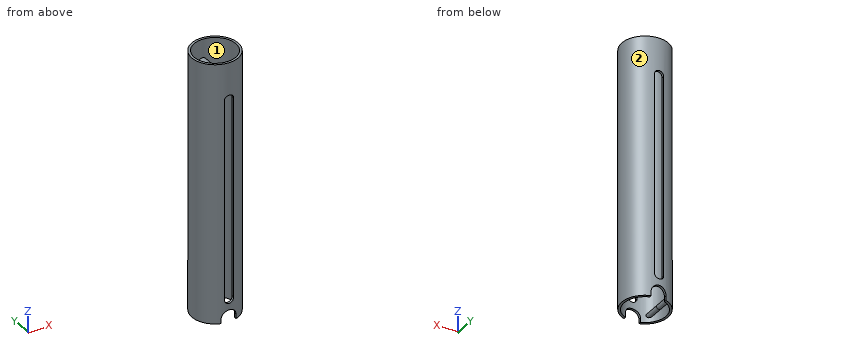
from build123d import *

# Parameters (mm, degrees)
ESQUISSE1_R                    = 5
ESQUISSE1_R_2                  = 4.5
BOSS_EXTRU_1_DEPTH             = 28
BOSS_EXTRU_2_REACH             = 7
ESQUISSE2_R                    = 1
ESQUISSE2_R_2                  = 0.5
BOSS_EXTRU_2_DIRECTION_2_REACH = 7
ENL_V_MAT_EXTRU_1_DEPTH        = 6
ENL_V_MAT_EXTRU_1_DEPTH_BACK   = 6
ENL_V_MAT_EXTRU_2_DEPTH        = 6.000000118
ENL_V_MAT_EXTRU_2_DEPTH_BACK   = 6.000000118


with BuildPart() as part:
    # Esquisse1 → Boss.-Extru.1 (new body, symmetric)
    with BuildSketch(Plane.XY):
        Circle(ESQUISSE1_R)
        Circle(ESQUISSE1_R_2, mode=Mode.SUBTRACT)
    extrude(amount=BOSS_EXTRU_1_DEPTH, both=True)

    # Esquisse2 → Boss.-Extru.2 (add, up to next)
    with BuildSketch(Plane(origin=(0, 0, 0), x_dir=(1, 0, 0), z_dir=(0, 1, 0)), mode=Mode.PRIVATE) as boss_extru_2_sk1:
        with Locations((0, -23)):
            Circle(ESQUISSE2_R)
    boss_extru_2_tool1 = extrude(boss_extru_2_sk1.sketch, amount=BOSS_EXTRU_2_REACH, mode=Mode.PRIVATE) - part.part
    add(boss_extru_2_tool1.solids().sort_by_distance((0, 0, 23))[0])
    # Esquisse2 → Boss.-Extru.2 (add, up to next)
    with BuildSketch(Plane(origin=(0, 0, 0), x_dir=(1, 0, 0), z_dir=(0, 1, 0)), mode=Mode.PRIVATE) as boss_extru_2_sk2:
        with Locations((-3, 26.5)):
            Circle(ESQUISSE2_R_2)
    boss_extru_2_tool2 = extrude(boss_extru_2_sk2.sketch, amount=BOSS_EXTRU_2_REACH, mode=Mode.PRIVATE) - part.part
    add(boss_extru_2_tool2.solids().sort_by_distance((-3, 0, -26.5))[0])

    # Esquisse2 → Boss.-Extru.2 direction 2 (add, up to next)
    with BuildSketch(Plane(origin=(0, 0, 0), x_dir=(1, 0, 0), z_dir=(0, 1, 0)), mode=Mode.PRIVATE) as boss_extru_2_direction_2_sk1:
        with Locations((0, -23)):
            Circle(ESQUISSE2_R)
    boss_extru_2_direction_2_tool1 = extrude(boss_extru_2_direction_2_sk1.sketch, amount=-BOSS_EXTRU_2_DIRECTION_2_REACH, mode=Mode.PRIVATE) - part.part
    add(boss_extru_2_direction_2_tool1.solids().sort_by_distance((0, 0, 23))[0])
    # Esquisse2 → Boss.-Extru.2 direction 2 (add, up to next)
    with BuildSketch(Plane(origin=(0, 0, 0), x_dir=(1, 0, 0), z_dir=(0, 1, 0)), mode=Mode.PRIVATE) as boss_extru_2_direction_2_sk2:
        with Locations((-3, 26.5)):
            Circle(ESQUISSE2_R_2)
    boss_extru_2_direction_2_tool2 = extrude(boss_extru_2_direction_2_sk2.sketch, amount=-BOSS_EXTRU_2_DIRECTION_2_REACH, mode=Mode.PRIVATE) - part.part
    add(boss_extru_2_direction_2_tool2.solids().sort_by_distance((-3, 0, -26.5))[0])

    # Esquisse3 → Enlèv. mat.-Extru.1 (cut, two sides)
    with BuildSketch(Plane(origin=(0, 0, 0), x_dir=(1, 0, 0), z_dir=(0, 1, 0))) as enl_v_mat_extru_1_sk:
        with BuildLine():
            Line((1, 23), (1, -20))
            ThreePointArc((1, -20), (0, -21), (-1, -20))
            Line((-1, -20), (-1, 23))
            ThreePointArc((-1, 23), (0, 24), (1, 23))
        make_face()
    extrude(amount=ENL_V_MAT_EXTRU_1_DEPTH, mode=Mode.SUBTRACT)
    extrude(enl_v_mat_extru_1_sk.sketch, amount=-ENL_V_MAT_EXTRU_1_DEPTH_BACK, mode=Mode.SUBTRACT)

    # Esquisse4 → Enlèv. mat.-Extru.2 (cut, two sides)
    with BuildSketch(Plane(origin=(0, 0, 0), x_dir=(1, 0, 0), z_dir=(0, 1, 0))) as enl_v_mat_extru_2_sk:
        with BuildLine():
            Line((-1.6, 27), (-1.6, 28))
            ThreePointArc((-1.6, 28), (0, 29.6), (1.6, 28))
            Line((1.6, 28), (1.6, 27))
            ThreePointArc((1.6, 27), (0, 25.4), (-1.6, 27))
        make_face()
    extrude(amount=ENL_V_MAT_EXTRU_2_DEPTH, mode=Mode.SUBTRACT)
    extrude(enl_v_mat_extru_2_sk.sketch, amount=-ENL_V_MAT_EXTRU_2_DEPTH_BACK, mode=Mode.SUBTRACT)


solid = part.part
Geometry check sheet. Reference: the model listing, model coordinates, mm. Face numbers are marked on the shaded views. Give positions to 0.01 mm unless a question says otherwise; leave off trailing zeros. Order: outer loops, then holes, each group sorted by start corner. A loop starts at its lowest first (then second) coordinate and runs counter-clockwise, first axis right, second up.
1) Cross-section at B-B (x = 0). Record the boundary of the cut face in (y, z).
Results are:
outline: (-5, -25.4) - (-4.5, -25.4) - (-4.5, -24) - (-5, -24) - close; (-5, 21) - (-4.5, 21) - (-4.5, 22) - (4.5, 22) - (4.5, 21) - (5, 21) - (5, 28) - (4.5, 28) - (4.5, 24) - (-4.5, 24) - (-4.5, 28) - (-5, 28) - close; (4.5, -25.4) - (5, -25.4) - (5, -24) - (4.5, -24) - close
2) Gauge pin test, flat ends, axial feed: pin 1 (1.5 mm diameter, centred on x = -2, z = 17.5, fed in from +Y); pin 2 (4 mm diameter, centred on x = -2.5, z = 1, fed in from -Y); pin 3 (1.5 mm diameter, centred on x = -3, y = -3, fed in from -Z). Record the tip position at first contact, or that the pin passes through.
Results are:
pin 1: stops at y = 4.84
pin 2: stops at y = -4.9
pin 3: stops at z = -28
3) Cross-section at D-D (y = -2). Record the boundary of the cut face in (x, z), then the cut area to 3 significant figures.
Results are:
outline: (-4.58, -28) - (-4.03, -28) - (-4.03, 28) - (-4.58, 28) - close; circle Ø1 at (-3, -26.5); circle Ø2 at (0, 23); (4.03, -28) - (4.58, -28) - (4.58, 28) - (4.03, 28) - close
area: 65.7 mm2
4) Cross-section at C-C (z = -26.5). Record the boundary of the cut face in (x, y), then the cut area to 3 significant figures.
Results are:
outline: (-2.5, -3.74) - (-2.5, 3.74) arc R4.5 cw to (-1.52, 4.24) - (-1.52, 4.76) arc R5 ccw to (-1.52, -4.76) - (-1.52, -4.24) arc R4.5 cw to start; (1.52, -4.76) arc R5 ccw to (1.52, 4.76) - (1.52, 4.24) arc R4.5 cw to (1.52, -4.24) - close; hole (-3.5, -2.83) - (-3.5, 2.83) arc R4.5 ccw to start
area: 18.5 mm2
5) Material ranges on probe 1 along Y at (x, z) = (2.5, 18.5); probe 2 along X at (y, z) = (0.25, -2); probe 3 along Y at (x, z) = (4, 16.5), recorded low to high.
Results are:
probe 1: y = -4.33 to -3.74, 3.74 to 4.33
probe 2: x = -4.99 to -4.49, 4.49 to 4.99
probe 3: y = -3 to -2.06, 2.06 to 3
6) Cross-section at A-A (z = 11). Record the boundary of the cut face in (x, y).
Results are:
outline: (-1, -4.9) - (-1, -4.39) arc R4.5 cw to (-1, 4.39) - (-1, 4.9) arc R5 ccw to start; (1, -4.9) arc R5 ccw to (1, 4.9) - (1, 4.39) arc R4.5 cw to (1, -4.39) - close
7) Draft check along Y on the marked faces 1 and 2. Enter one of: released by +Y, released by -Y, zero draft, split by the parting line, or undercut.
Results are:
face 1: undercut
face 2: split by the parting line
